Here's how the part is built. I have some questions about the finished solid (model axes, mm). A direction names the side the tool comes from. Give positions to 0.01 mm unless a question says otherwise; leave off trailing zeros. Write each loop counter-clockwise with the first axis right and the second up, starting at its lowest first coordinate (ties: lowest second). Pieces come first, ordered by that corner, then holes. Notation, with made-up numbers: (-27.5, 16) -> (10.5, 16) arc R15 cw to (10.5, 41) -> close; hole circle Ø3 at (89, -39.5). An arc over 180 degrees is marked (long way). Use CSV: the item, a comma, the result in double quotes. Start each with the question number.
(1) Suppose I cut it at A-A on x = 29. List the corners of the cut face in (y, z) for me, plus the area to 4 significant figures.
(2) I need wall thicknesses on L1, parallel to Y at x = 0, z = 3; L2, parallel to Z at x = 42, y = 15; L3, parallel to X at y = -4, z = 7.25. Which ranges of each line are inside material? Lowest first, please. Write a range as [from, to].
(3) Which directions (+Z, -Z, +X, -X, +Y, -Y) give clear straight access to the entire face, cutting with the end or side of a thin tool? Please do faces 4 (the cylindrical face through (12.693, -7.864, 2.782)), 5 (the conical face through (-28.6, -15.43, 0.36)), 6 (the conical face through (-36.655, -25.858, 13.464)), 7 (the cylindrical face through (-36.281, -0.357, 13.595)).
(4) Suppose I cut it at B-B on y = 9. Give the number of separate pieces and of enclosed holes in the cut face, plus the area to 3 significant figures.
(5) For pin 1 Ø3 at (y, z) = (9.5, 8.5) entering from +X; pin 2 Ø4 at (y, z) = (-10, 12.5) entering from -X; pin 3 Ø3 at (y, z) = (14.5, 14) entering from -X, each with a flat end and sliding along its axis, tell me the tip position at first contact or that it passes through.
(6) If we mould it in two halves opening along X, with no side actions, what happens to faces 1 (the cylindrical face through (-46.246, -0.357, 8.187)), 2 (the flat face through (0, 26, 4)), 3 (the flat face through (-50, 0, 4))? For each: pulls with the +X half, pulls with the -X half, needs draft (parallel to the pull), parting line crosses it, or undercut.
Autodesk Fusion 360 part; units mm, degrees
sketch "Sketch1" plane through (0, 0, 0) normal (0, 0, 1) x (1, 0, 0)
  line L0 (50, -26) -> (-50, -26)
  line L1 (-50, -26) -> (-50, 26)
  line L2 (-50, 26) -> (50, 26)
  line L3 (50, 26) -> (50, -26)
  line L4 (50, -26) -> (-50, 26) construction
  line L5 (-50, -26) -> (50, 26) construction
  line L6 (-34, 26) -> (-34, -26)
  line L7 (34, 26) -> (34, -26)
  line L8 (24, 22) -> (34, 22)
  line L9 (34, 22) -> (34, -22)
  line L10 (34, -22) -> (24, -22)
  line L11 (24, -22) -> (24, 22)
  line L12 (-24, 11) -> (16, 11)
  line L13 (16, 11) -> (16, -11)
  line L14 (16, -11) -> (-24, -11)
  line L15 (-24, -11) -> (-24, 11)
  line L16 (50, 0) -> (-34, 0) construction
  line L17 (-29, 18.5) -> (21, 18.5)
  line L18 (21, 18.5) -> (21, 15)
  line L19 (21, 15) -> (-29, 15)
  line L20 (-29, 15) -> (-29, 18.5)
  line L21 (-4, -11) -> (-4, 41) construction
  line L22 (-29, -18.5) -> (21, -18.5)
  line L23 (21, -15) -> (-29, -15)
  line L24 (-29, -15) -> (-29, -18.5)
  line L25 (21, -18.5) -> (21, -15)
  dimension "d15" = 52
  dimension "d16" = 16
  dimension "d17" = 16
  dimension "d18" = 10
  dimension "d19" = 44
  dimension "d22" = 100
  dimension "d23" = 10
  dimension "d24" = 40
  dimension "d25" = 22
  dimension "d26" = 11
  dimension "d27" = 3.5
  dimension "d28" = 4
  dimension "d29" = 50
extrude "Extrude1" add sketch "Sketch1" along normal blind 5 contours L0 L2 L3 L7 L9 | L0 L2 L6 L7 L8 L10 L11 | L0 L1 L2 L6
extrude "Extrude2" add sketch "Sketch1" along normal blind 16 contours L0 L2 L3 L7 L9 | L0 L1 L2 L6
fillet "Fillet1" radius 11 4 edges at (-24, -11, 2.5) (16, -11, 2.5) (16, 11, 2.5) (-24, 11, 2.5)
fillet "Fillet2" radius 8 4 edges at (-50, 0, 16) (-34, 0, 16) (34, 0, 16) (50, 0, 16)
fillet "Fillet3" radius 1.75 8 edges at (-29, 18.5, 2.5) (-29, -15, 2.5) (21, 18.5, 2.5) (21, -15, 2.5) (21, -18.5, 2.5) (21, 15, 2.5) (-29, -18.5, 2.5) (-29, 15, 2.5)
sketch "Sketch2" plane through (0, -26, 0) normal (0, -1, 0) x (1, 0, 0)
  arc A0 (50, 8) -> (34, 8) centre (42, 8) ccw
  line L0 (34, 8) -> (34, 5)
  line L1 (34, 5) -> (-34, 5)
  line L2 (-34, 5) -> (-34, 8)
  arc A1 (-34, 8) -> (-50, 8) centre (-42, 8) ccw
  line L3 (-50, 8) -> (-50, 0)
  line L4 (-50, 0) -> (50, 0)
  line L5 (50, 0) -> (50, 8)
  circle A2 centre (-42, 8) radius 4.25
  circle A3 centre (42, 8) radius 4.25
  dimension "d40" = 8.5
  dimension "d41" = 8.5
extrude "Extrude3" cut sketch "Sketch2" against normal blind 55 contours A2 | A3
chamfer "Chamfer1" distance 0.5 angle 45 18 edges at (-50, 0, 0) (50, 0, 0) (0, -26, 0) (-45.9624, -26, 9.5369) (38.0376, -26, 9.5369) (0, 26, 5) (0, -26, 5) (42, -26, 16) (50, -26, 4) (34, -26, 6.5) (-42, -26, 16) (-34, -26, 6.5) (-50, -26, 4) (50, 26, 4) (42, 26, 16) (34, 26, 6.5) (38.0376, 26, 6.4631) (-45.9624, 26, 6.4631) 5 faces at (50, -8.6667, 5.3344) (42.7619, -8.6667, 15.9638) (34, 7.3333, 1.6667) (-41.3333, 0.0007, 0) (-11.3333, 26, 1.6667)
equation "d26 = d25 / 2"
equation "d40 = draadstang"
equation "d41 = d40"
equation "draadstang = 8.5 mm"
Geometry says:
1,outline,"(-26, 0.5) -> (-25.5, 0) -> (-22.5, 0) -> (-22, 0.5) -> (-22, 5) -> (-25.5, 5) -> (-26, 4.5) -> close; (22, 0.5) -> (22.5, 0) -> (25.5, 0) -> (26, 0.5) -> (26, 4.5) -> (25.5, 5) -> (22, 5) -> close"
1,area,"39.25 mm²"
2,L1,"[-26, -18.5], [-15, -11], [11, 15], [18.5, 26]"
2,L2,"[0, 3.75], [12.25, 16]"
2,L3,"[-50, -46.18], [-37.82, -34], [34, 37.82], [46.18, 50]"
3,face 4,"+Z, -Z"
3,face 5,"-Z"
3,face 6,"+Z, -Y"
3,face 7,"+Z, +Y, -Y"
4,separate pieces,"3"
4,enclosed holes,"2"
4,area,"479 mm²"
5,pin 1,"x = 50"
5,pin 2,"x = -49.6"
5,pin 3,"x = -48.62"
6,face 1,"undercut"
6,face 2,"needs draft"
6,face 3,"pulls with the -X half"
